Check sheet for the modelled part. Datum: model origin and axes. Units: mm. A direction names the side the tool comes from. Give positions to 0.01 mm unless a question says otherwise; leave off trailing zeros. Write each loop counter-clockwise with the first axis right and the second up, starting at its lowest first coordinate (ties: lowest second). Pieces come first, ordered by that corner, then holes.
from build123d import *

# Parameters (mm, degrees)
F0_R     = 26.7
F0_R_2   = 24.7
F1_DEPTH = 50
F2_R     = 26.7
F3_DEPTH = 3
F4_R     = 31.7
F4_R_2   = 26.7
F4_R_3   = 24.7
F5_DEPTH = 3


with BuildPart() as f1:
    # F0 (on Top) → F1 (new body)
    with BuildSketch(Plane.XY):
        Circle(F0_R)
        Circle(F0_R_2, mode=Mode.SUBTRACT)
    extrude(amount=F1_DEPTH)

    # F2 (on face) → F3 (join)
    with BuildSketch(Plane.XY.offset(50)):
        Circle(F2_R)
    extrude(amount=F3_DEPTH)

    # F4 (on face) → F5 (join)
    with BuildSketch(Plane(origin=(0, 0, 0), x_dir=(1, 0, 0), z_dir=(0, 0, -1))):
        Circle(F4_R)
        Circle(F4_R_2, mode=Mode.SUBTRACT)
        Circle(F4_R_2)
        Circle(F4_R_3, mode=Mode.SUBTRACT)
    extrude(amount=-F5_DEPTH)


solid = f1.part
1) Sectioned sample at A-A on y = 0. Record the boundary of the cut face in (x, z).
2) Draft check along Y on faces 4 (the flat face through (-17, 21, 3)), 5 (the cylindrical face through (30.236, -9.522, 1.479)), 6 (the cylindrical face through (23.56, 7.42, 24.65)). Enter one of: +Y half, -Y half, draft (parallel to the pull), parting line (faces both ways), or undercut.
3) Gauge pin test, flat ends, axial feed: pin 1 (1 mm diameter, centred on y = 24.5, z = 17.5, fed in from -X); pin 2 (10 mm diameter, centred on x = 2, z = 33, fed in from -Y); pin 3 (3 mm diameter, centred on x = -2, z = 22.5, fed in from +Y). Record the tip position at first contact, or that the pin passes through.
4) Sectioned sample at C-C on z = 9. Record the boundary of the cut face in (x, y), then the cut area to 3 significant figures.
5) Scan lines: L1, parallel to Y at x = 0, z = 21; L2, parallel to Z at x = -3, y = 22.5; L3, parallel to Z at x = 8.5, y = -27. Record each from-to range of solid material in increasing order.
6) Access from +Z, -Z, +X, -X, +Y, -Y to the whole of each face (thin tool, end or side, straight path). Record for faces 1 (the flat face through (-17, 19, 0)), 2 (the cylindrical face through (25.467, 8.02, 27.65)), 3 (the flat face through (0, 0, 50)).
Answers below:
1. outline: (-31.7, 0) - (-24.7, 0) - (-24.7, 50) - (24.7, 50) - (24.7, 0) - (31.7, 0) - (31.7, 3) - (26.7, 3) - (26.7, 53) - (-26.7, 53) - (-26.7, 3) - (-31.7, 3) - close
2. face 4: draft
2. face 5: parting line
2. face 6: undercut
3. pin 1: stops at x = -11.7
3. pin 2: stops at y = -26.7
3. pin 3: stops at y = 26.7
4. outline: circle Ø53.4 at (0, 0); hole circle Ø49.4 at (0, 0)
4. area: 323 mm2
5. L1: y = -26.7 to -24.7, 24.7 to 26.7
5. L2: z = 50 to 53
5. L3: z = 0 to 3
6. face 1: -Z, +X, -X, +Y, -Y
6. face 2: +Z
6. face 3: -Z
